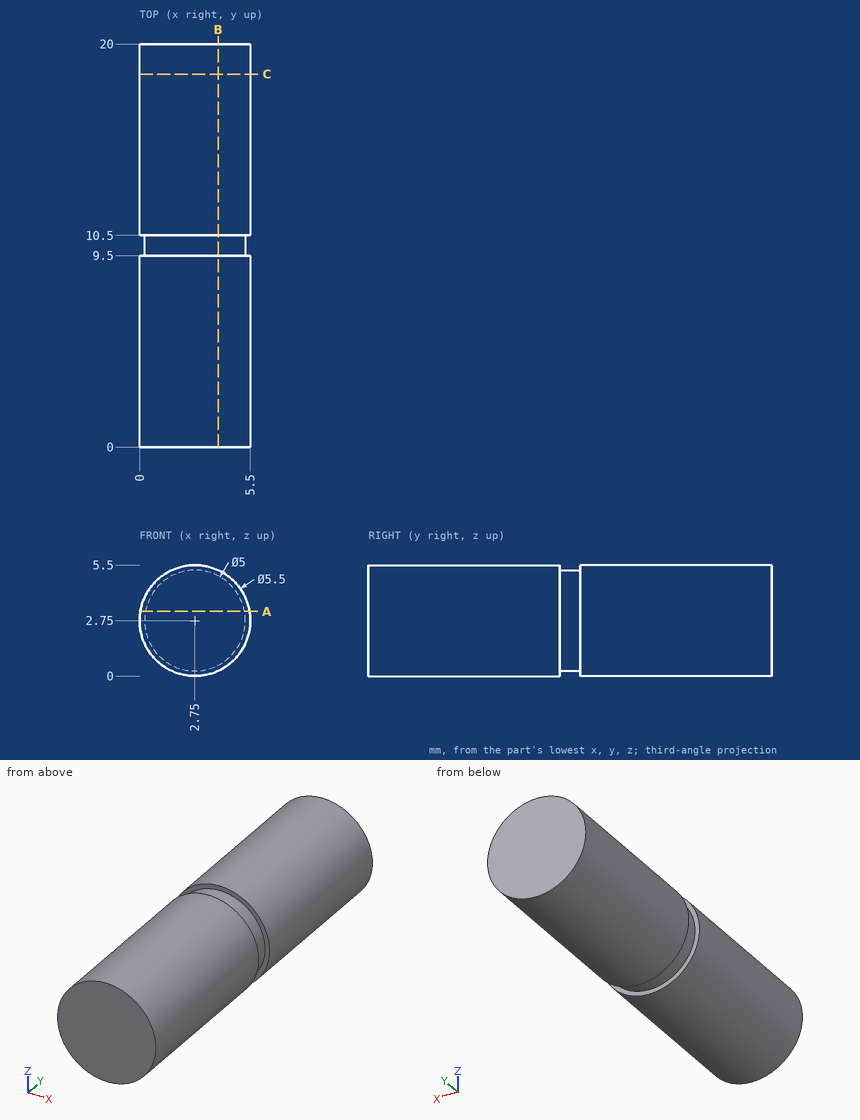
Check sheet for the drawn part. Datum: minimum x, y, z corner. Units: mm. Round coordinates to 2 decimals unless told otherwise and drop trailing zeros. Order: outer loops, then holes, each group sorted by start corner. A loop starts at its lowest first (then second) coordinate and runs counter-clockwise, first axis right, second up.
1) Section check C-C (y = 18.5). Record the boundary of the cut face in (x, z), and give its area (3 significant figures).
2) Section check B-B (x = 3.9). Record the boundary of the cut face in (y, z), and give its area (3 significant figures).
3) Section check A-A (z = 3.2). Record the boundary of the cut face in (x, y).
4) Scan lines: line 1 (X direction, y = 11.5, z = 2.85); line 2 (X direction, y = 8.5, z = 3.9). Record each from-to range of solid material in increasing order.
Result:
1. outline: circle Ø5.5 at (2.75, 2.75)
1. area: 23.8 mm2
2. outline: (0, 0.25) - (9.5, 0.25) - (9.5, 0.53) - (10.5, 0.53) - (10.5, 0.25) - (20, 0.25) - (20, 5.25) - (10.5, 5.25) - (10.5, 4.97) - (9.5, 4.97) - (9.5, 5.25) - (0, 5.25) - close
2. area: 99.4 mm2
3. outline: (0.04, 0) - (5.46, 0) - (5.46, 9.5) - (5.21, 9.5) - (5.21, 10.5) - (5.46, 10.5) - (5.46, 20) - (0.04, 20) - (0.04, 10.5) - (0.29, 10.5) - (0.29, 9.5) - (0.04, 9.5) - close
4. line 1: x = 0 to 5.5
4. line 2: x = 0.25 to 5.25
